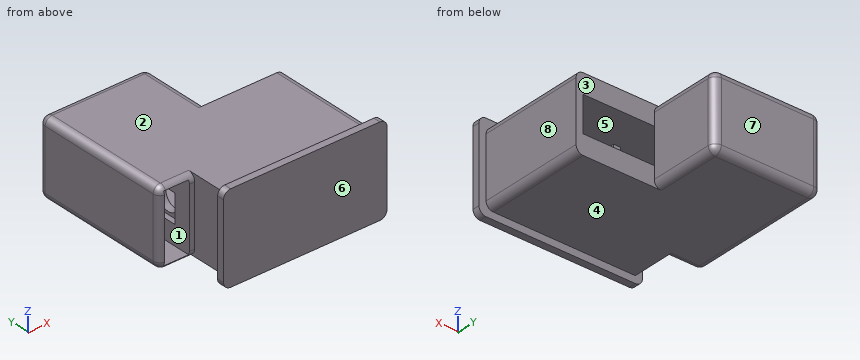
from build123d import *

# Parameters (mm, degrees)
SKETCH2_W               = 210
SKETCH2_H               = 105
SKETCH2_W_2             = 190
SKETCH2_H_2             = 50
BOSS_EXTRUDE2_DEPTH     = 150
FILLET3_R               = 10
FILLET4_R               = 10
SKETCH4_W               = 230
SKETCH4_H               = 125
BOSS_EXTRUDE3_DEPTH     = 10
FILLET5_R               = 10
FILLET6_R               = 10
FILLET7_R               = 10
FILLET8_R               = 10
SKETCH7_W               = 10
SKETCH7_H               = 50
BOSS_EXTRUDE4_DEPTH     = 93.9
SKETCH8_R               = 16.1
CUT_EXTRUDE2_DEPTH      = 10
SKETCH10_R              = 16.1
CUT_EXTRUDE3_DEPTH      = 10
SKETCH14_W              = 150
SKETCH14_H              = 105
BOSS_EXTRUDE6_DEPTH     = 100
CUT_EXTRUDE4_DEPTH      = 1
CUT_EXTRUDE4_DEPTH_BACK = 145
SKETCH19_W              = 95
SKETCH19_H              = 90
SKETCH22_W              = 50
SKETCH22_H              = 105
SKETCH22_W_2            = 35
SKETCH22_H_2            = 95
BOSS_EXTRUDE7_DEPTH     = 100
SKETCH24_W              = 40
SKETCH24_H              = 40
CUT_EXTRUDE5_DEPTH      = 10
SKETCH25_W              = 95.055428317
SKETCH25_H              = 90
BOSS_EXTRUDE9_DEPTH     = 5
FILLET9_R               = 10
FILLET10_R              = 10
FILLET11_R              = 10
FILLET12_R              = 10
FILLET13_R              = 10
FILLET15_R              = 10
SKETCH28_W              = 35
SKETCH28_H              = 95
CUT_EXTRUDE7_DEPTH      = 5


with BuildPart() as part:
    # Sketch2 → Boss-Extrude2 (new body)
    with BuildSketch(Plane(origin=(0, 0, 0), x_dir=(1, 0, 0), z_dir=(0, 1, 0))):
        Rectangle(SKETCH2_W, SKETCH2_H)
        Rectangle(SKETCH2_W_2, SKETCH2_H_2, mode=Mode.SUBTRACT)
    extrude(amount=BOSS_EXTRUDE2_DEPTH)

    # Fillet3
    fillet3_edges = [part.edges().sort_by_distance(p)[0] for p in [
        (105, 75, 52.5),
    ]]
    fillet(fillet3_edges, radius=FILLET3_R)

    # Fillet4
    fillet4_edges = [part.edges().sort_by_distance(p)[0] for p in [
        (105, 75, -52.5),
    ]]
    fillet(fillet4_edges, radius=FILLET4_R)

    # Sketch4 → Boss-Extrude3 (add)
    with BuildSketch(Plane(origin=(0, 0, 0), x_dir=(1, 0, 0), z_dir=(0, 1, 0))):
        Rectangle(SKETCH4_W, SKETCH4_H)
    extrude(amount=-BOSS_EXTRUDE3_DEPTH)

    # Fillet5
    fillet5_edges = [part.edges().sort_by_distance(p)[0] for p in [
        (115, -5, 62.5),
    ]]
    fillet(fillet5_edges, radius=FILLET5_R)

    # Fillet6
    fillet6_edges = [part.edges().sort_by_distance(p)[0] for p in [
        (115, -5, -62.5),
    ]]
    fillet(fillet6_edges, radius=FILLET6_R)

    # Fillet7
    fillet7_edges = [part.edges().sort_by_distance(p)[0] for p in [
        (-115, -5, -62.5),
    ]]
    fillet(fillet7_edges, radius=FILLET7_R)

    # Fillet8
    fillet8_edges = [part.edges().sort_by_distance(p)[0] for p in [
        (-115, -5, 62.5),
    ]]
    fillet(fillet8_edges, radius=FILLET8_R)

    # Sketch7 → Boss-Extrude4 (add)
    with BuildSketch(Plane(origin=(0, 0, 0), x_dir=(1, 0, 0), z_dir=(0, 1, 0))):
        Rectangle(SKETCH7_W, SKETCH7_H)
    extrude(amount=BOSS_EXTRUDE4_DEPTH)

    # Sketch8 → Cut-Extrude2 (cut)
    with BuildSketch(Plane.ZY.offset(5)):
        with Locations((0, 93.9)):
            Circle(SKETCH8_R)
    extrude(amount=-CUT_EXTRUDE2_DEPTH, mode=Mode.SUBTRACT)

    # Sketch10 → Cut-Extrude3 (cut)
    with BuildSketch(Plane.ZY.offset(105)):
        with Locations((0.019819576, 93.900003501)):
            Circle(SKETCH10_R)
    extrude(amount=-CUT_EXTRUDE3_DEPTH, mode=Mode.SUBTRACT)

    # Sketch14 → Boss-Extrude6 (add)
    with BuildSketch(Plane(origin=(0, 150, 0), x_dir=(1, 0, 0), z_dir=(0, 1, 0))):
        with Locations((-80, 0)):
            Rectangle(SKETCH14_W, SKETCH14_H)
    extrude(amount=BOSS_EXTRUDE6_DEPTH)

    # Sketch19 → Cut-Extrude4 (cut, two sides: drawn at the far end of the back side and taken through both)
    with BuildSketch(Plane.ZY.offset(155).offset(-CUT_EXTRUDE4_DEPTH_BACK)):
        with Locations((0, 200)):
            Rectangle(SKETCH19_W, SKETCH19_H)
    extrude(amount=CUT_EXTRUDE4_DEPTH + CUT_EXTRUDE4_DEPTH_BACK, mode=Mode.SUBTRACT)

    # Sketch22 → Boss-Extrude7 (add)
    with BuildSketch(Plane.XZ.offset(-150)):
        with Locations((-130, 0)):
            Rectangle(SKETCH22_W, SKETCH22_H)
        with Locations((-130, 0)):
            Rectangle(SKETCH22_W_2, SKETCH22_H_2, mode=Mode.SUBTRACT)
    extrude(amount=BOSS_EXTRUDE7_DEPTH)

    # Sketch24 → Cut-Extrude5 (cut)
    with BuildSketch(Plane(origin=(-105, 0, 0), x_dir=(0, 0, -1), z_dir=(1, 0, 0))):
        with Locations((-0.019819576, 93.900003501)):
            Rectangle(SKETCH24_W, SKETCH24_H)
    extrude(amount=-CUT_EXTRUDE5_DEPTH, mode=Mode.SUBTRACT)

    # Sketch25 → Boss-Extrude9 (add)
    with BuildSketch(Plane.ZY.offset(155)):
        with Locations((0.027714159, 200)):
            Rectangle(SKETCH25_W, SKETCH25_H)
    extrude(amount=-BOSS_EXTRUDE9_DEPTH)

    # Fillet9
    fillet9_edges = [part.edges().sort_by_distance(p)[0] for p in [
        (-80, 250, -52.5),
        (-155, 250, 0),
        (-80, 250, 52.5),
        (-5, 250, 0),
    ]]
    fillet(fillet9_edges, radius=FILLET9_R)

    # Fillet10
    # the kernel refuses this fillet: 10 mm, written as the material it takes off along each edge
    with BuildSketch(Plane(origin=(-145, 240, 42.5), x_dir=(-1, 0, 0), z_dir=(0, 0, 1))) as fillet10_piece_1_section:
        Polygon((0, 0), (FILLET10_R, 0), (FILLET10_R, -FILLET10_R), (0, -FILLET10_R), align=None)
    fillet10_piece_1 = extrude(amount=FILLET10_R, mode=Mode.PRIVATE)
    fillet10_piece_1 = fillet10_piece_1 - Plane(origin=(-145, 240, 42.5), x_dir=(0.7071067811865475, -0.7071067811865475, 0), z_dir=(0, 0, 1)) * Sphere(FILLET10_R, mode=Mode.PRIVATE)
    add(fillet10_piece_1, mode=Mode.SUBTRACT)
    with BuildSketch(Plane(origin=(-155, 240, 52.5), x_dir=(1, 0, 0), z_dir=(0, -1, 0))) as fillet10_piece_2:
        with BuildLine():
            CenterArc((FILLET10_R, -FILLET10_R), FILLET10_R, 90, 90)
            Line((0, -FILLET10_R), (0, 0))
            Line((0, 0), (FILLET10_R, 0))
        make_face()
    extrude(amount=215, mode=Mode.SUBTRACT)

    # Fillet11
    # the kernel refuses this fillet: 10 mm, written as the material it takes off along each edge
    with BuildSketch(Plane(origin=(-145, 240, -42.5), x_dir=(-1, 0, 0), z_dir=(0, 0, -1))) as fillet11_piece_1_section:
        Polygon((0, 0), (FILLET11_R, 0), (FILLET11_R, FILLET11_R), (0, FILLET11_R), align=None)
    fillet11_piece_1 = extrude(amount=FILLET11_R, mode=Mode.PRIVATE)
    fillet11_piece_1 = fillet11_piece_1 - Plane(origin=(-145, 240, -42.5), x_dir=(0.7071067811865475, -0.7071067811865475, 0), z_dir=(0, 0, -1)) * Sphere(FILLET11_R, mode=Mode.PRIVATE)
    add(fillet11_piece_1, mode=Mode.SUBTRACT)
    with BuildSketch(Plane(origin=(-155, 25, -52.5), x_dir=(1, 0, 0), z_dir=(0, 1, 0))) as fillet11_piece_2:
        with BuildLine():
            CenterArc((FILLET11_R, -FILLET11_R), FILLET11_R, 90, 90)
            Line((0, -FILLET11_R), (0, 0))
            Line((0, 0), (FILLET11_R, 0))
        make_face()
    extrude(amount=215, mode=Mode.SUBTRACT)

    # Fillet12
    # the kernel refuses this fillet: 10 mm, written as the material it takes off along each edge
    with BuildSketch(Plane(origin=(-15, 240, 42.5), x_dir=(1, 0, 0), z_dir=(0, 0, 1))) as fillet12_piece_1_section:
        Polygon((0, 0), (FILLET12_R, 0), (FILLET12_R, FILLET12_R), (0, FILLET12_R), align=None)
    fillet12_piece_1 = extrude(amount=FILLET12_R, mode=Mode.PRIVATE)
    fillet12_piece_1 = fillet12_piece_1 - Plane(origin=(-15, 240, 42.5), x_dir=(-0.7071067811865475, -0.7071067811865475, 0), z_dir=(0, 0, 1)) * Sphere(FILLET12_R, mode=Mode.PRIVATE)
    add(fillet12_piece_1, mode=Mode.SUBTRACT)
    with BuildSketch(Plane(origin=(-5, 150, 52.5), x_dir=(-1, 0, 0), z_dir=(0, 1, 0))) as fillet12_piece_2:
        with BuildLine():
            CenterArc((FILLET12_R, -FILLET12_R), FILLET12_R, 90, 90)
            Line((0, -FILLET12_R), (0, 0))
            Line((0, 0), (FILLET12_R, 0))
        make_face()
    extrude(amount=90, mode=Mode.SUBTRACT)

    # Fillet13
    # the kernel refuses this fillet: 10 mm, written as the material it takes off along each edge
    with BuildSketch(Plane(origin=(-15, 240, -42.5), x_dir=(1, 0, 0), z_dir=(0, 0, -1))) as fillet13_piece_1_section:
        Polygon((0, 0), (FILLET13_R, 0), (FILLET13_R, -FILLET13_R), (0, -FILLET13_R), align=None)
    fillet13_piece_1 = extrude(amount=FILLET13_R, mode=Mode.PRIVATE)
    fillet13_piece_1 = fillet13_piece_1 - Plane(origin=(-15, 240, -42.5), x_dir=(-0.7071067811865475, -0.7071067811865475, 0), z_dir=(0, 0, -1)) * Sphere(FILLET13_R, mode=Mode.PRIVATE)
    add(fillet13_piece_1, mode=Mode.SUBTRACT)
    with BuildSketch(Plane(origin=(-5, 150, -52.5), x_dir=(-1, 0, 0), z_dir=(0, 1, 0))) as fillet13_piece_2:
        with BuildLine():
            CenterArc((FILLET13_R, FILLET13_R), FILLET13_R, 180, 90)
            Line((0, FILLET13_R), (0, 0))
            Line((0, 0), (FILLET13_R, 0))
        make_face()
    extrude(amount=90, mode=Mode.SUBTRACT)

    # Fillet15
    # the kernel refuses this fillet: 10 mm, written as the material it takes off along each edge
    with BuildSketch(Plane(origin=(-145, 50, 52.5), x_dir=(0, 1, 0), z_dir=(1, 0, 0)), Plane(origin=(-105, 50, -52.5), x_dir=(0, 1, 0), z_dir=(-1, 0, 0))) as fillet15_piece_1:
        with BuildLine():
            CenterArc((FILLET15_R, -FILLET15_R), FILLET15_R, 90, 90)
            Line((0, -FILLET15_R), (0, 0))
            Line((0, 0), (FILLET15_R, 0))
        make_face()
    extrude(amount=40, mode=Mode.SUBTRACT)
    with BuildSketch(Plane(origin=(-155, 50, -42.5), x_dir=(0, 1, 0), z_dir=(0, 0, 1))) as fillet15_piece_2:
        with BuildLine():
            CenterArc((FILLET15_R, -FILLET15_R), FILLET15_R, 90, 90)
            Line((0, -FILLET15_R), (0, 0))
            Line((0, 0), (FILLET15_R, 0))
        make_face()
    extrude(amount=85, mode=Mode.SUBTRACT)
    with BuildSketch(Plane(origin=(-145, 50, 42.5), x_dir=(-1, 0, 0), z_dir=(0, 0, -1))) as fillet15_piece_3:
        with BuildLine():
            CenterArc((10 - FILLET15_R, FILLET15_R), FILLET15_R, 270, 90)
            Line((10, FILLET15_R), (10, 0))
            Line((10, 0), (10 - FILLET15_R, 0))
        make_face()
    revolve(axis=Axis((-145, 50, 42.5), (0, 1, 0)), revolution_arc=90, mode=Mode.SUBTRACT)
    with BuildSketch(Plane(origin=(-145, 50, -42.5), x_dir=(-1, 0, 0), z_dir=(0, 0, 1))) as fillet15_piece_4:
        with BuildLine():
            CenterArc((10 - FILLET15_R, -FILLET15_R), FILLET15_R, 0, 90)
            Line((10 - FILLET15_R, 0), (10, 0))
            Line((10, 0), (10, -FILLET15_R))
        make_face()
    revolve(axis=Axis((-145, 50, -42.5), (0, -1, 0)), revolution_arc=90, mode=Mode.SUBTRACT)

    # Sketch28 → Cut-Extrude7 (cut)
    with BuildSketch(Plane.XZ.offset(-150)):
        with Locations((-130, 0)):
            Rectangle(SKETCH28_W, SKETCH28_H)
    extrude(amount=-CUT_EXTRUDE7_DEPTH, mode=Mode.SUBTRACT)


solid = part.part
Input: part model. Units: mm. Frame: model coordinates. Face numbers are marked on the shaded views. A direction names the side the tool comes from. Round coordinates to 2 decimals unless told otherwise and drop trailing zeros. Loops run counter-clockwise (first coordinate to the right, second up) from the corner with the lowest first, then second, coordinate; pieces in that order, holes last. Notation, with made-up numbers: (-8, -25.5) -> (15, -25.5) arc R22 cw to (15, -17.5) -> close; hole circle Ø9 at (-32, 16). An arc over 180 degrees is marked (long way). Answer as a JSON object with one key per item and string values. Group by question number.
1) Pin query (flat end, axial travel): pin 1 (2.5 mm diameter, centred on x = 1.5, z = 20, fed in from +Y); pin 2 (5 mm diameter, centred on x = -98.5, y = 77.5, fed in from +Z); pin 3 (1.5 mm diameter, centred on x = -10.5, y = 77, fed in from -Z). Return the tip coordinate at first contact, or that it passes through.
2) Section query B-B on x = -56.5. Output: boundary loops of the cut face in (y, z).
3) Section query D-D on y = 221. Output: boundary loops of the cut face in (x, z).
4) Section query C-C on x = 27. Output: boundary loops of the cut face in (y, z), plus the area to 3 significant figures.
5) Ray query, L1, parallel to Y at x = -42, z = 10; L2, parallel to Z at x = -18.5, y = 194; L3, parallel to X at y = 114, z = 21. Return the intervals inside material, ascending.
6) Reachability of the marked faces 4, 5, 6, 7 and 8 from +Z, -Z, +X, -X, +Y, -Y: full face, straight path, thin tool, end or side. Return the list, or none.
7) Section query A-A on y = 143. Output: boundary loops of the cut face in (x, z), plus the area to 3 significant figures.
8) Draft query along Z for the marked faces 1, 2 and 3. Return one class per face: +Z half, -Z half, draft (parallel to the pull), parting line (faces both ways), or undercut.
Reply:
{
 "1": {"pin 1": "stops at y = 93.9", "pin 2": "stops at z = 52.5", "pin 3": "stops at z = -52.5"},
 "2": {"outline": "(-10, -62.5) -> (0, -62.5) -> (0, -52.5) -> (240, -52.5) arc R10 ccw to (250, -42.5) -> (250, 42.5) arc R10 ccw to (240, 52.5) -> (0, 52.5) -> (0, 62.5) -> (-10, 62.5) -> close; hole (0, -25) -> (150, -25) -> (150, 25) -> (0, 25) -> close; hole (155, -47.5) -> (245, -47.5) -> (245, 47.5) -> (155, 47.5) -> close"},
 "3": {"outline": "(-155, -42.5) arc R10 ccw to (-145, -52.5) -> (-15, -52.5) arc R10 ccw to (-5, -42.5) -> (-5, 42.5) arc R10 ccw to (-15, 52.5) -> (-145, 52.5) arc R10 ccw to (-155, 42.5) -> close; hole (-150, -47.5) -> (-10, -47.5) -> (-10, 47.5) -> (-150, 47.5) -> close"},
 "4": {"outline": "(-10, -62.5) -> (0, -62.5) -> (0, -52.5) -> (150, -52.5) -> (150, -25) -> (0, -25) -> (0, 25) -> (150, 25) -> (150, 52.5) -> (0, 52.5) -> (0, 62.5) -> (-10, 62.5) -> close", "area": "9,500 mm2"},
 "5": {"L1": "y = -10 to 0, 150 to 155, 245 to 250", "L2": "z = -52.5 to -47.5, 47.5 to 52.5", "L3": "x = -155 to -147.5, -112.5 to -95, 95 to 105"},
 "6": {"face 4": "-Z, +X, -X, +Y", "face 5": "none", "face 6": "+Z, -Z, +X, -X, -Y", "face 7": "+Z, -Z, +X, -X, +Y", "face 8": "+Z, -Z, +X, +Y"},
 "7": {"outline": "(-155, -42.5) arc R10 ccw to (-145, -52.5) -> (95, -52.5) arc R10 ccw to (105, -42.5) -> (105, 42.5) arc R10 ccw to (95, 52.5) -> (-145, 52.5) arc R10 ccw to (-155, 42.5) -> close; hole (-147.5, -47.5) -> (-112.5, -47.5) -> (-112.5, 47.5) -> (-147.5, 47.5) -> close; hole (-95, -25) -> (95, -25) -> (95, 25) -> (-95, 25) -> close", "area": "14,400 mm2"},
 "8": {"face 1": "undercut", "face 2": "+Z half", "face 3": "draft"}
}
